Autodesk Inventor part; units mm, degrees
ref_plane "YZ Plane" through (0, 0, 0) normal (1, 0, 0) x (0, 1, 0)
ref_plane "XZ Plane" through (0, 0, 0) normal (0, 1, 0) x (-1, 0, 0)
ref_plane "XY Plane" through (0, 0, 0) normal (0, 0, 1) x (1, 0, 0)
sketch "Sketch1" plane through (0, 0, 0) normal (0, 0, 1) x (1, 0, 0)
  point P0 (0, 0)
sketch "0" plane through (0, 0, 0) normal (0, 0, 1) x (1, 0, 0)
  line L0 (-20.32, 48.26) -> (-5.08, 48.26)
  line L1 (-5.08, 48.26) -> (-5.08, 42.672)
  line L2 (-5.08, 42.672) -> (-20.32, 42.672)
  line L3 (-20.32, 42.672) -> (-20.32, 48.26)
  line L4 (-36.95, -0.635) -> (-36.95, 4.953)
  line L5 (-36.95, 4.953) -> (-51.95, 4.953)
  line L6 (-51.95, 4.953) -> (-51.95, -0.635)
  line L7 (-51.95, -0.635) -> (-36.95, -0.635)
  line L8 (-20.32, -0.635) -> (-5.08, -0.635)
  line L9 (-5.08, -0.635) -> (-5.08, 4.953)
  line L10 (-5.08, 4.953) -> (-20.32, 4.953)
  line L11 (-20.32, 4.953) -> (-20.32, -0.635)
  line L12 (-60.96, 54.61) -> (-60.96, -3.81)
  line L13 (-60.96, -3.81) -> (3.81, -3.81)
  line L14 (3.81, -3.81) -> (3.81, 54.61)
  line L15 (3.81, 54.61) -> (-60.96, 54.61)
  line L16 (-60.96, -3.81) -> (3.81, -3.81)
  line L17 (3.81, -3.81) -> (3.81, 54.61)
  line L18 (-60.96, 54.61) -> (-60.96, -3.81)
  line L19 (-60.96, -3.81) -> (3.81, -3.81)
  line L20 (-50.8, 28.956) -> (-38.12, 28.956)
  line L21 (-38.12, 28.956) -> (-38.12, 34.544)
  line L22 (-38.12, 34.544) -> (-50.8, 34.544)
  line L23 (-50.8, 34.544) -> (-50.8, 28.956)
  line L24 (-44.45, 31.75) -> (-50.8, 31.75)
  line L25 (-50.8, 31.75) -> (-50.8, 28.956)
  line L26 (-50.8, 28.956) -> (-44.45, 28.956)
  line L27 (-44.45, 28.956) -> (-44.45, 31.75)
  line L28 (-20.32, 0.3568) -> (-36.95, 0.3568)
  line L29 (-50.8, 54.61) -> (-60.96, 54.61)
  line L30 (-5.08, -3.81) -> (3.81, -3.81)
  line L31 (3.81, -3.81) -> (3.81, 54.61)
  circle A0 centre (-54.61, 31.75) radius 1.0922
  circle A1 centre (-34.29, 31.75) radius 1.0922
  line L32 (-54.61, 31.75) -> (-34.29, 31.75)
  line L33 (3.81, 55.118) -> (-60.96, 55.118)
  line L34 (-60.96, -4.318) -> (3.81, -4.318)
  line L35 (-60.96, 55.118) -> (3.81, 55.118)
  line L36 (3.81, 55.118) -> (3.81, -4.318)
  line L37 (3.81, -4.318) -> (-60.96, -4.318)
  line L38 (-60.96, -4.318) -> (-60.96, 55.118)
  line L39 (-60.96, 58.293) -> (6.985, 58.293)
  line L40 (6.985, 58.293) -> (6.985, -4.318)
  line L41 (-64.135, 55.118) -> (-64.135, -7.493)
  line L42 (-64.135, -7.493) -> (3.81, -7.493)
  line L43 (-64.135, 55.118) -> (-60.96, 55.118)
  line L44 (-60.96, 55.118) -> (-60.96, 58.293)
  line L45 (-60.96, 58.293) -> (-64.135, 58.293)
  line L46 (-64.135, 58.293) -> (-64.135, 55.118)
  line L47 (6.985, -4.318) -> (3.81, -4.318)
  line L48 (3.81, -4.318) -> (3.81, -7.493)
  line L49 (3.81, -7.493) -> (6.985, -7.493)
  line L50 (6.985, -7.493) -> (6.985, -4.318)
  line L51 (-20.32, 2.8338) -> (-5.08, 2.8338)
  line L52 (-5.08, 2.8338) -> (-5.08, 8.5488)
  line L53 (-5.08, 8.5488) -> (-20.32, 8.5488)
  line L54 (-20.32, 8.5488) -> (-20.32, 2.8338)
  line L55 (-51.95, 0.3568) -> (-36.95, 0.3568)
  line L56 (-36.95, 0.3568) -> (-36.95, 5.832)
  line L57 (-36.95, 5.832) -> (-51.95, 5.832)
  line L58 (-51.95, 5.832) -> (-51.95, 0.3568)
  point P0 (-20.32, 51.435)
  point P1 (-5.08, 48.26)
  point P2 (-5.08, 42.672)
  point P3 (-20.32, 45.847)
  dimension "d0" = 0.508
  dimension "d1" = 0.508
  dimension "d2" = 3.175
  dimension "d3" = 3.175
  dimension "d9" = 15.24
  dimension "d10" = 5.588
  dimension "d11" = 90
  dimension "d13" = 5.588
  dimension "d14" = 5.588
  dimension "d15" = 15.24
  dimension "d16" = 15.24
  dimension "d17" = 6.35
  dimension "d18" = 5.715
extrude "Extrusion1" add sketch "0" along normal blind 3.175 contours L7 L6 L55 L4 | L11 L51 L9 L8 | L15 L14 L13 L12 | L38 L33 L36 L15 | L12 L38 L34 L48 L42 L41 L43 | L13 L36 L34 L38 | L44 L39 L40 L47 L36 L14 L33 | L43 L46 L45 L44 | L47 L50 L49 L48 | A0 | A1
sketch "Sketch3" plane through (0, 0, 0) normal (0, 0, -1) x (-1, 0, 0)
  line L0 (-6.985, -7.493) -> (-6.985, 58.293)
  line L1 (64.135, -7.493) -> (-6.985, -7.493)
  line L2 (64.135, 58.293) -> (64.135, -7.493)
  line L3 (-6.985, 58.293) -> (64.135, 58.293)
  line L4 (36.95, 5.832) -> (36.95, 0.3568)
  line L5 (51.95, 0.3568) -> (51.95, 5.832)
  line L6 (50.8, 28.956) -> (50.8, 34.544)
  line L7 (38.12, 28.956) -> (50.8, 28.956)
  line L8 (38.12, 34.544) -> (38.12, 28.956)
  line L9 (50.8, 34.544) -> (38.12, 34.544)
  line L10 (20.32, 2.8338) -> (20.32, 8.5488)
  line L11 (5.08, 8.5488) -> (5.08, 2.8338)
  line L12 (-3.81, 55.118) -> (-3.81, -4.318)
  line L13 (-3.81, -4.318) -> (60.96, -4.318)
  line L14 (60.96, -4.318) -> (60.96, 55.118)
  line L15 (60.96, 55.118) -> (-3.81, 55.118)
  line L16 (5.08, 2.8338) -> (20.32, 2.8338)
  line L17 (20.32, 8.5488) -> (5.08, 8.5488)
  line L18 (36.95, 0.3568) -> (51.95, 0.3568)
  line L19 (51.95, 5.832) -> (36.95, 5.832)
  point P0 (0, 0)
  dimension "d6" = 3.175
extrude "Extrusion2" add sketch "Sketch3" along normal blind 8.89 contours L0 L3 L2 L1
properties part number "pololuAndRelayCaseTop" material "Rubber, Silicone"
Could you check a few things on this model? Use its own coordinates, in mm. A direction names the side the tool comes from. Coordinates: 2 decimals unless noted, no trailing zeros. Write each loop counter-clockwise with the first axis right and the second up, starting at its lowest first coordinate (ties: lowest second). Pieces come first, ordered by that corner, then holes. Notation, with made-up numbers: M 65,-25 L 78,-25 A18 ccw 78,7 Z; hole C -17,70 d1. An arc over 180 degrees is marked long. Answer as CSV lines item,"result". Start each with the question number.
1) For P1, Ø2, axis at x = -53.5, y = 6.5, coming from the -Z side, with a flat end and sliding along its axis, tell me the tip position at first contact or that it passes through.
2) I want a section at D-D, the plane x = -1.5. Please give me the cut outline in (y, z) (3 decimals).
3) I want a section at A-A, the plane x = -10.5. Please give me the cut outline in (y, z) (3 decimals).
4) For faces 4 (the flat face through (-13, 8.549, 2)), 5 (the flat face through (-29, 26, 3.175)), 6 (the flat face through (-29, 26, 0)), which set-ups out of +Z, -Z, +X, -X, +Y, -Y let a thin tool reach every point of the face, with its end or its side?
5) I want a section at C-C, the plane y = 45. Please give me the cut outline in (x, z) (3 decimals), and give its area (3 significant figures).
6) Please list where these lines run through material, in increasing order: line 1 (X direction, y = 21.5, z = -7.5) (3 decimals); line 2 (Y direction, x = -40.5, z = 1); line 3 (Y direction, x = -21, z = -3). Write a range as from..to.
7) I want a section at B-B, the plane z = 1.25. Please give me the cut outline in (x, y) (3 decimals), and give its area (3 significant figures).
8) We'd pull the mould along Y, two halves only. Please class faces 1 (the flat face through (-38.12, 32, 2)), 2 (the flat face through (-26, -6, -8.89)), 3 (the flat face through (-28, 58.293, -3)): +Y half, -Y half, draft (parallel to the pull), parting line (faces both ways), or undercut.
Data:
1,P1,"stops at z = 0"
2,outline,"M -7.493,-8.89 L -4.318,-8.89 L -4.318,0 L 55.118,0 L 55.118,-8.89 L 58.293,-8.89 L 58.293,3.175 L -7.493,3.175 Z"
3,outline,"M -7.493,-8.89 L -4.318,-8.89 L -4.318,0 L 2.834,0 L 2.834,3.175 L -7.493,3.175 Z; M 8.549,0 L 42.672,0 L 42.672,3.175 L 8.549,3.175 Z; M 48.26,0 L 55.118,0 L 55.118,-8.89 L 58.293,-8.89 L 58.293,3.175 L 48.26,3.175 Z"
4,face 4,"+Z, -Z"
4,face 5,"+Z, +X, -X, +Y, -Y"
4,face 6,"-Z"
5,outline,"M -64.135,-8.89 L -60.96,-8.89 L -60.96,0 L -20.32,0 L -20.32,3.175 L -64.135,3.175 Z; M -5.08,0 L 3.81,0 L 3.81,-8.89 L 6.985,-8.89 L 6.985,3.175 L -5.08,3.175 Z"
5,area,"234 mm^2"
6,line 1,"x = -64.135..-60.96, 3.81..6.985"
6,line 2,"y = -7.49..0.36, 5.83..28.96, 34.54..58.29"
6,line 3,"y = -7.49..-4.32, 55.12..58.29"
7,outline,"M -64.135,-7.493 L 6.985,-7.493 L 6.985,58.293 L -64.135,58.293 Z; hole M -51.95,0.357 L -36.95,0.357 L -36.95,5.832 L -51.95,5.832 Z; hole M -50.8,28.956 L -38.12,28.956 L -38.12,34.544 L -50.8,34.544 Z; hole M -20.32,2.834 L -5.08,2.834 L -5.08,8.549 L -20.32,8.549 Z; hole M -20.32,42.672 L -5.08,42.672 L -5.08,48.26 L -20.32,48.26 Z"
7,area,"4,350 mm^2"
8,face 1,"undercut"
8,face 2,"draft"
8,face 3,"+Y half"
